```python
from build123d import *

# Parameters (mm, degrees)
SKETCH1_W                  = 330.2
SKETCH1_H                  = 38.1
BOSS_EXTRUDE1_DEPTH        = 2.38125
F_10_START                 = -2.38125
F_10_CLEARANCE_SLOT1_DEPTH = 4.7625
F_1_4_20_TAPPED_HOLE1_D    = 5.7912


# Read off the part's stored shape, not the designer's step: #10 Clearance Slot1
with BuildPart() as part:
    # Sketch1 → Boss-Extrude1 (new, symmetric)
    with BuildSketch(Plane(origin=(0, 0, 0), x_dir=(1, 0, 0), z_dir=(0, 1, 0))):
        Rectangle(SKETCH1_W, SKETCH1_H)
    extrude(amount=BOSS_EXTRUDE1_DEPTH, both=True)

    # #10 Clearance Slot1 outline → #10 Clearance Slot1 (cut)
    with BuildSketch(Plane(origin=(0, 0, 0), x_dir=(1, 0, 0), z_dir=(0, 1, 0)).offset(F_10_START)):
        with BuildLine():
            Line((142.2527, 10.1473), (149.8473, 10.1473))
            ThreePointArc((149.8473, 10.1473), (152.4, 12.7), (149.8473, 15.2527))
            Line((149.8473, 15.2527), (142.2527, 15.2527))
            ThreePointArc((142.2527, 15.2527), (139.7, 12.7), (142.2527, 10.1473))
        make_face()
        with BuildLine():
            ThreePointArc((105.3973, 10.1473), (107.95, 12.7), (105.3973, 15.2527))
            Line((105.3973, 15.2527), (97.8027, 15.2527))
            ThreePointArc((97.8027, 15.2527), (95.25, 12.7), (97.8027, 10.1473))
            Line((97.8027, 10.1473), (105.3973, 10.1473))
        make_face()
        with BuildLine():
            ThreePointArc((-142.2527, 10.1473), (-139.7, 12.7), (-142.2527, 15.2527))
            Line((-142.2527, 15.2527), (-149.8473, 15.2527))
            ThreePointArc((-149.8473, 15.2527), (-152.4, 12.7), (-149.8473, 10.1473))
            Line((-149.8473, 10.1473), (-142.2527, 10.1473))
        make_face()
        with BuildLine():
            ThreePointArc((-97.8027, 10.1473), (-95.25, 12.7), (-97.8027, 15.2527))
            Line((-97.8027, 15.2527), (-105.3973, 15.2527))
            ThreePointArc((-105.3973, 15.2527), (-107.95, 12.7), (-105.3973, 10.1473))
            Line((-105.3973, 10.1473), (-97.8027, 10.1473))
        make_face()
        with BuildLine():
            Line((142.2527, -15.2527), (149.8473, -15.2527))
            ThreePointArc((149.8473, -15.2527), (152.4, -12.7), (149.8473, -10.1473))
            Line((149.8473, -10.1473), (142.2527, -10.1473))
            ThreePointArc((142.2527, -10.1473), (139.7, -12.7), (142.2527, -15.2527))
        make_face()
        with BuildLine():
            ThreePointArc((105.3973, -15.2527), (107.95, -12.7), (105.3973, -10.1473))
            Line((105.3973, -10.1473), (97.8027, -10.1473))
            ThreePointArc((97.8027, -10.1473), (95.25, -12.7), (97.8027, -15.2527))
            Line((97.8027, -15.2527), (105.3973, -15.2527))
        make_face()
        with BuildLine():
            ThreePointArc((-97.8027, -15.2527), (-95.25, -12.7), (-97.8027, -10.1473))
            Line((-97.8027, -10.1473), (-105.3973, -10.1473))
            ThreePointArc((-105.3973, -10.1473), (-107.95, -12.7), (-105.3973, -15.2527))
            Line((-105.3973, -15.2527), (-97.8027, -15.2527))
        make_face()
        with BuildLine():
            ThreePointArc((-142.2527, -15.2527), (-139.7, -12.7), (-142.2527, -10.1473))
            Line((-142.2527, -10.1473), (-149.8473, -10.1473))
            ThreePointArc((-149.8473, -10.1473), (-152.4, -12.7), (-149.8473, -15.2527))
            Line((-149.8473, -15.2527), (-142.2527, -15.2527))
        make_face()
    extrude(amount=F_10_CLEARANCE_SLOT1_DEPTH, mode=Mode.SUBTRACT)

    # 1/4-20 Tapped Hole1 (through all)
    with Locations(Plane(origin=(0, 2.38125, 0), x_dir=(1, 0, 0), z_dir=(0, 1, 0))):
        with Locations((-50.8, 9.525), (-50.8, -9.525), (50.8, -9.525), (50.8, 9.525)):
            Hole(F_1_4_20_TAPPED_HOLE1_D / 2)


solid = part.part
```
CAD build for the part. Positions are in the model's coordinates, mm. Give positions to 0.01 mm unless a question says otherwise; leave off trailing zeros. Loops run counter-clockwise (first coordinate to the right, second up) from the corner with the lowest first, then second, coordinate; pieces in that order, holes last. Notation, with made-up numbers: (50.5, 62) -> (84.5, 62) arc R13 ccw to (84.5, 78) -> close; hole circle Ø7 at (78, 25). An arc over 180 degrees is marked (long way). Use a Markdown table: item, result.
1. Mould opens along Z. For faces 1 (the flat face through (-2, 2.381, 0)), 2 (the cylindrical face through (53.693, -0.033, 9.398)) say: pulls with the +Z half, pulls with the -Z half, needs draft (parallel to the pull), parting line crosses it, or undercut.
Check result:
| item | result |
|---|---|
| face 1 | needs draft |
| face 2 | undercut |
2. Slice it at A-A (x = -50.8). List the corners of the cut face in (y, z), plus the area to 3 significant figures.
Check result:
| item | result |
|---|---|
| outline | (-2.38, -19.05) -> (2.38, -19.05) -> (2.38, -12.42) -> (-2.38, -12.42) -> close; (-2.38, -6.63) -> (2.38, -6.63) -> (2.38, 6.63) -> (-2.38, 6.63) -> close; (-2.38, 12.42) -> (2.38, 12.42) -> (2.38, 19.05) -> (-2.38, 19.05) -> close |
| area | 126 mm^2 |
3. Wall check: L1, parallel to Z at x = 50.8, y = 0.9; L2, parallel to X at y = -0.7, z = -12.5; L3, parallel to X at y = -0.7, z = 13.5. Give the ranges that are in metal, low to high. Write a range as [from, to].
Check result:
| item | result |
|---|---|
| L1 | z = [-19.05, -12.42], [-6.63, 6.63], [12.42, 19.05] |
| L2 | x = [-165.1, -152.39], [-139.71, -107.94], [-95.26, 95.26], [107.94, 139.71], [152.39, 165.1] |
| L3 | x = [-165.1, -152.27], [-139.83, -107.82], [-95.38, 95.38], [107.82, 139.83], [152.27, 165.1] |
4. Slice it at B-B (y = -0.85). Give the number of separate pieces and of enclosed holes in the cut face, plus the area to 3 significant figures.
Check result:
| item | result |
|---|---|
| separate pieces | 1 |
| enclosed holes | 12 |
| area | 12,000 mm^2 |
